Can you work these out from the model? Positions are in its coordinate system, mm. Give positions to 0.01 mm unless a question says otherwise; leave off trailing zeros. Write each loop counter-clockwise with the first axis right and the second up, starting at its lowest first coordinate (ties: lowest second). Pieces come first, ordered by that corner, then holes. Notation, with made-up numbers: (-13, 28.25) - (33, 28.25) arc R23 ccw to (33, 54.25) - close; hole circle Ø11 at (12.5, 58). An arc over 180 degrees is marked (long way). Return JSON: item names as keys, results as strings. Group by question number.
from build123d import *

# Parameters (mm, degrees)
F0_R     = 1
F1_DEPTH = 1
F2_R     = 5.08
F3_R     = 5.08
F4_R     = 5.08
F5_R     = 5.08


with BuildPart() as f1:
    # F0 (on Top) → F1 (new body)
    with BuildSketch(Plane.XY):
        with BuildLine():
            Line((0, 22), (0, 0))
            Line((0, 0), (0, -22))
            Line((0, -22), (14.035148, -34))
            Line((14.035148, -34), (27.999999, -34))
            Line((27.999999, -34), (27.999999, -22))
            Line((27.999999, -22), (57.999999, -22))
            Line((57.999999, -22), (57.999999, -34))
            Line((57.999999, -34), (67.999999, -34))
            ThreePointArc((67.999999, -34), (87.562333, -27.808544), (100, -11.489123))
            Line((100, -11.489123), (100, 11.489123))
            ThreePointArc((100, 11.489123), (87.562333, 27.808544), (67.999999, 34))
            Line((67.999999, 34), (57.999999, 34))
            Line((57.999999, 34), (57.999999, 22))
            Line((57.999999, 22), (27.999999, 22))
            Line((27.999999, 22), (27.999999, 34))
            Line((27.999999, 34), (14.035148, 34))
            Line((14.035148, 34), (0, 22))
        make_face()
        with Locations((21.140715, -20)):
            Circle(F0_R, mode=Mode.SUBTRACT)
        with Locations((43.140715, -20)):
            Circle(F0_R, mode=Mode.SUBTRACT)
        with Locations((21.140715, 20)):
            Circle(F0_R, mode=Mode.SUBTRACT)
        with Locations((43.140715, 20)):
            Circle(F0_R, mode=Mode.SUBTRACT)
    extrude(amount=F1_DEPTH)

    # F2
    f2_edges = [f1.edges().sort_by_distance(p)[0] for p in [
        (14.035148, 34, 0.5),
    ]]
    fillet(f2_edges, radius=F2_R)

    # F3
    f3_edges = [f1.edges().sort_by_distance(p)[0] for p in [
        (0, 22, 0.5),
    ]]
    fillet(f3_edges, radius=F3_R)

    # F4
    f4_edges = [f1.edges().sort_by_distance(p)[0] for p in [
        (0, -22, 0.5),
    ]]
    fillet(f4_edges, radius=F4_R)

    # F5
    f5_edges = [f1.edges().sort_by_distance(p)[0] for p in [
        (14.035148, -34, 0.5),
    ]]
    fillet(f5_edges, radius=F5_R)


solid = f1.part
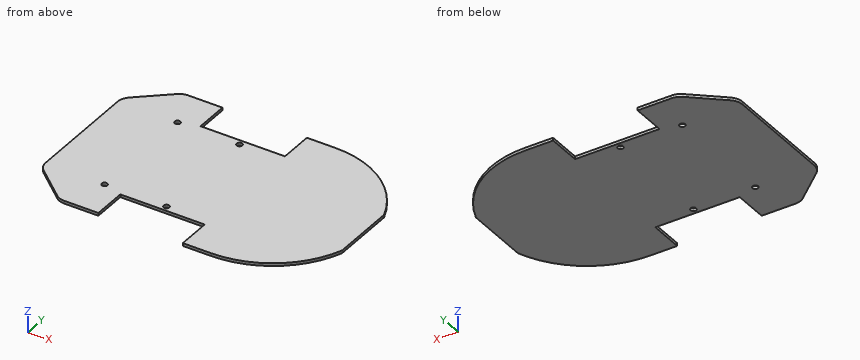
1) Imagine slicing it at D-D, the plane x = 85. Write out the boundary of the cut face in (y, z), and give its area (3 significant figures).
2) Imagine slicing it at A-A, the plane z = 0.65. Write out the boundary of the cut face in (x, y).
3) Will these pins go through, and if not, where does the flat tip stop? pin 1 Ø0.5 at (x, z) = (43.5, 0.5) entering from +Y; pin 2 Ø1.6 at (x, y) = (43.14, -20) entering from -Z; pin 3 Ø0.5 at (y, z) = (-25, 0.5) entering from +X.
4) Imagine slicing it at B-B, the plane y = 27. Write out the boundary of the cut face in (x, z), and give its area (3 significant figures).
5) I need wall thicknesses on line 1 along Y through (x, z) = (21, 0.5); line 2 along X through (y, z) = (-13.5, 0.1); line 3 along Y through (x, z) = (76, 0.55). Which ranges of each line are inside material? Lowest first, please.
6) Imagine slicing it at C-C, the plane x = 38. Write out the boundary of the cut face in (y, z), and give its area (3 significant figures).
Resolved:
{
 "1": {"outline": "(-29.44, 0) - (29.44, 0) - (29.44, 1) - (-29.44, 1) - close", "area": "58.9 mm^2"},
 "2": {"outline": "(0, -19.66) arc R5.08 ccw to (1.78, -23.52) - (12.61, -32.78) arc R5.08 ccw to (15.91, -34) - (28, -34) - (28, -22) - (58, -22) - (58, -34) - (68, -34) arc R34 ccw to (100, -11.49) - (100, 11.49) arc R34 ccw to (68, 34) - (58, 34) - (58, 22) - (28, 22) - (28, 34) - (15.91, 34) arc R5.08 ccw to (12.61, 32.78) - (1.78, 23.52) arc R5.08 ccw to (0, 19.66) - close; hole circle Ø2 at (21.14, -20); hole circle Ø2 at (21.14, 20); hole circle Ø2 at (43.14, -20); hole circle Ø2 at (43.14, 20)"},
 "3": {"pin 1": "y = 22", "pin 2": "through", "pin 3": "x = 91.31"},
 "4": {"outline": "(5.85, 0) - (28, 0) - (28, 1) - (5.85, 1) - close; (58, 0) - (88.66, 0) - (88.66, 1) - (58, 1) - close", "area": "52.8 mm^2"},
 "5": {"line 1": "-34 to -20.99, -19.01 to 19.01, 20.99 to 34", "line 2": "0 to 99.2", "line 3": "-33.05 to 33.05"},
 "6": {"outline": "(-22, 0) - (22, 0) - (22, 1) - (-22, 1) - close", "area": "44.0 mm^2"}
}
